Check sheet for the modelled part. Datum: model origin and axes. Units: mm. Give positions to 0.01 mm unless a question says otherwise; leave off trailing zeros. Order: outer loops, then holes, each group sorted by start corner. A loop starts at its lowest first (then second) coordinate and runs counter-clockwise, first axis right, second up.
from build123d import *

# Parameters (mm, degrees)
F0_W     = 25
F0_H     = 10
F0_R     = 2
F1_DEPTH = 7.5
F2_R     = 2


# Not quite as in the source:
# - a feature names something its author has since deleted; it is built from what else it names


with BuildPart() as f1:
    # F0 (on Top) → F1 (new body, symmetric)
    with BuildSketch(Plane.XY):
        Polygon((17.8516533444, 33), (20.875, 33), (20.8, 33.6), (17.7766533444, 33.6), align=None)
        Polygon((17.7766533444, 33.6), (20.8, 33.6), (20.3125, 37.5), (17.2891533444, 37.5), align=None)
        Polygon((17.2891533444, 37.5), (20.3125, 37.5), (20.2375, 38.1), (17.2141533444, 38.1), align=None)
        Polygon((17.2141533444, 38.1), (20.2375, 38.1), (19.75, 42), (16.7266533444, 42), align=None)
        Polygon((16.7266533444, 42), (19.75, 42), (19.675, 42.6), (16.6516533444, 42.6), align=None)
        Polygon((16.6516533444, 42.6), (19.675, 42.6), (19.1875, 46.5), (16.1641533444, 46.5), align=None)
        Polygon((16.1641533444, 46.5), (19.1875, 46.5), (19.1125, 47.1), (16.0891533444, 47.1), align=None)
        Polygon((16.0891533444, 47.1), (19.1125, 47.1), (18.625, 51), (15.6016533444, 51), align=None)
        Polygon((15.6016533444, 51), (18.625, 51), (18.55, 51.6), (15.5266533444, 51.6), align=None)
        Polygon((15.5266533444, 51.6), (18.55, 51.6), (18.0625, 55.5), (15.0391533444, 55.5), align=None)
        Polygon((15.0391533444, 55.5), (18.0625, 55.5), (17.9875, 56.1), (14.9641533444, 56.1), align=None)
        Polygon((14.9641533444, 56.1), (17.9875, 56.1), (17.5, 60), (14.4766533444, 60), align=None)
        Polygon((14.4766533444, 60), (17.5, 60), (17.425, 60.6), (14.4016533444, 60.6), align=None)
        Polygon((14.4016533444, 60.6), (17.425, 60.6), (16.9375, 64.5), (13.9141533444, 64.5), align=None)
        Polygon((13.9141533444, 64.5), (16.9375, 64.5), (16.8625, 65.1), (13.8391533444, 65.1), align=None)
        Polygon((13.8391533444, 65.1), (16.8625, 65.1), (16.375, 69), (13.3516533444, 69), align=None)
        Polygon((13.3516533444, 69), (16.375, 69), (16.3, 69.6), (13.2766533444, 69.6), align=None)
        Polygon((12.5, 100), (8.7, 69.6), (11.7233466556, 69.6), (12.5, 75.8132267551), (13.2766533444, 69.6), (16.3, 69.6), align=None)
        with Locations((12.5, -5)):
            Rectangle(F0_W, F0_H)
        with Locations((5, -5)):
            Circle(F0_R, mode=Mode.SUBTRACT)
        with Locations((20, -5)):
            Circle(F0_R, mode=Mode.SUBTRACT)
        Polygon((8.0625, 64.5), (7.575, 60.6), (10.5983466556, 60.6), (11.0858466556, 64.5), align=None)
        Polygon((8.7, 69.6), (8.625, 69), (11.6483466556, 69), (11.7233466556, 69.6), align=None)
        Polygon((8.1375, 65.1), (8.0625, 64.5), (11.0858466556, 64.5), (11.1608466556, 65.1), align=None)
        Polygon((8.625, 69), (8.1375, 65.1), (11.1608466556, 65.1), (11.6483466556, 69), align=None)
        Polygon((6.375, 51), (5.8875, 47.1), (8.9108466556, 47.1), (9.3983466556, 51), align=None)
        Polygon((7.5, 60), (7.0125, 56.1), (10.0358466556, 56.1), (10.5233466556, 60), align=None)
        Polygon((7.0125, 56.1), (6.9375, 55.5), (9.9608466556, 55.5), (10.0358466556, 56.1), align=None)
        Polygon((7.575, 60.6), (7.5, 60), (10.5233466556, 60), (10.5983466556, 60.6), align=None)
        Polygon((6.45, 51.6), (6.375, 51), (9.3983466556, 51), (9.4733466556, 51.6), align=None)
        Polygon((6.9375, 55.5), (6.45, 51.6), (9.4733466556, 51.6), (9.9608466556, 55.5), align=None)
        Polygon((5.25, 42), (4.7625, 38.1), (7.7858466556, 38.1), (8.2733466556, 42), align=None)
        Polygon((4.2, 33.6), (4.125, 33), (7.1483466556, 33), (7.2233466556, 33.6), align=None)
        Polygon((5.325, 42.6), (5.25, 42), (8.2733466556, 42), (8.3483466556, 42.6), align=None)
        Polygon((5.8125, 46.5), (5.325, 42.6), (8.3483466556, 42.6), (8.8358466556, 46.5), align=None)
        Polygon((4.6875, 37.5), (4.2, 33.6), (7.2233466556, 33.6), (7.7108466556, 37.5), align=None)
        Polygon((4.125, 33), (0, 0), (25, 0), (20.875, 33), (17.8516533444, 33), (18.3391533444, 29.1), (18.4141533444, 28.5), (18.9016533444, 24.6), (18.9766533444, 24), (19.4641533444, 20.1), (19.5391533444, 19.5), (20.0266533444, 15.6), (20.1016533444, 15), (20.5891533444, 11.1), (20.6641533444, 10.5), (21.1516533444, 6.6), (21.2266533444, 6), (21.6016533444, 3), (3.3983466556, 3), (3.7733466556, 6), (3.8483466556, 6.6), (4.3358466556, 10.5), (4.4108466556, 11.1), (4.8983466556, 15), (4.9733466556, 15.6), (5.4608466556, 19.5), (5.5358466556, 20.1), (6.0233466556, 24), (6.0983466556, 24.6), (6.5858466556, 28.5), (6.6608466556, 29.1), (7.1483466556, 33), align=None)
        Polygon((5.8875, 47.1), (5.8125, 46.5), (8.8358466556, 46.5), (8.9108466556, 47.1), align=None)
        Polygon((4.7625, 38.1), (4.6875, 37.5), (7.7108466556, 37.5), (7.7858466556, 38.1), align=None)
        Polygon((21.1516533444, 6.6), (3.8483466556, 6.6), (3.7733466556, 6), (21.2266533444, 6), align=None)
        Polygon((20.5891533444, 11.1), (4.4108466556, 11.1), (4.3358466556, 10.5), (20.6641533444, 10.5), align=None)
        Polygon((20.0266533444, 15.6), (4.9733466556, 15.6), (4.8983466556, 15), (20.1016533444, 15), align=None)
        Polygon((19.4641533444, 20.1), (5.5358466556, 20.1), (5.4608466556, 19.5), (19.5391533444, 19.5), align=None)
        Polygon((18.9016533444, 24.6), (6.0983466556, 24.6), (6.0233466556, 24), (18.9766533444, 24), align=None)
        Polygon((18.3391533444, 29.1), (6.6608466556, 29.1), (6.5858466556, 28.5), (18.4141533444, 28.5), align=None)
        Polygon((7.2233466556, 33.6), (7.1483466556, 33), (17.8516533444, 33), (17.7766533444, 33.6), align=None)
        Polygon((7.7858466556, 38.1), (7.7108466556, 37.5), (17.2891533444, 37.5), (17.2141533444, 38.1), align=None)
        Polygon((8.3483466556, 42.6), (8.2733466556, 42), (16.7266533444, 42), (16.6516533444, 42.6), align=None)
        Polygon((8.9108466556, 47.1), (8.8358466556, 46.5), (16.1641533444, 46.5), (16.0891533444, 47.1), align=None)
        Polygon((9.4733466556, 51.6), (9.3983466556, 51), (15.6016533444, 51), (15.5266533444, 51.6), align=None)
        Polygon((10.0358466556, 56.1), (9.9608466556, 55.5), (15.0391533444, 55.5), (14.9641533444, 56.1), align=None)
        Polygon((10.5983466556, 60.6), (10.5233466556, 60), (14.4766533444, 60), (14.4016533444, 60.6), align=None)
        Polygon((11.1608466556, 65.1), (11.0858466556, 64.5), (13.9141533444, 64.5), (13.8391533444, 65.1), align=None)
        Polygon((11.7233466556, 69.6), (11.6483466556, 69), (13.3516533444, 69), (13.2766533444, 69.6), align=None)
    extrude(amount=F1_DEPTH, both=True)

    # F2
    f2_edges = [f1.edges().sort_by_distance(p)[0] for p in [
        (12.5, 100, 0),
    ]]
    fillet(f2_edges, radius=F2_R)


solid = f1.part
1) Section check A-A, the plane y = -5. Record the cut outline in (x, z).
Recorded:
outline: (0, -7.5) - (3, -7.5) - (3, 7.5) - (0, 7.5) - close; (7, -7.5) - (18, -7.5) - (18, 7.5) - (7, 7.5) - close; (22, -7.5) - (25, -7.5) - (25, 7.5) - (22, 7.5) - close
2) Material ranges on L1, parallel to X at y = 30.5, z = 6.5; L2, parallel to X at y = 12.5, z = 4.5; L3, parallel to X at y = 20, z = 5.25, recorded low to high.
Recorded:
L1: x = 3.81 to 6.84, 18.16 to 21.19
L2: x = 1.56 to 4.59, 20.41 to 23.44
L3: x = 2.5 to 22.5
3) Depth check by flat-ended pin: pin 1 Ø3 at (y, z) = (62, 1.5) entering from +X; pin 2 Ø7.5 at (x, z) = (9.5, 2.5) entering from +Y; pin 3 Ø3 at (x, y) = (14, 17.5) entering from -Z; pin 4 Ø1.5 at (y, z) = (17, -5.5) entering from -X. Enter the tip coordinate at first touch or a pass-through.
Recorded:
pin 1: stops at x = 17.44
pin 2: stops at y = 85.88
pin 3: passes through
pin 4: stops at x = 2.03
4) Section check D-D, the plane x = 2. Record the cut outline in (y, z), then the cut area to 3 significant figures.
Recorded:
outline: (-10, -7.5) - (16, -7.5) - (16, 7.5) - (-10, 7.5) - close
area: 390 mm2
5) Section check C-C, the plane z = -5. State how many separate pieces and enclosed holes the cut face has, then the cut area to 3 significant figures.
Recorded:
separate pieces: 1
enclosed holes: 18
area: 871 mm2
6) Section check B-B, the plane y = 74.5. Record the cut outline in (x, z), then the cut area to 3 significant figures.
Recorded:
outline: (9.31, -7.5) - (12.34, -7.5) - (12.34, 7.5) - (9.31, 7.5) - close; (12.66, -7.5) - (15.69, -7.5) - (15.69, 7.5) - (12.66, 7.5) - close
area: 90.7 mm2
